from build123d import *

# Parameters (mm, degrees)
ESQUISSE7_R                  = 2.05
BOSS_EXTRU_1_DEPTH           = 8
ESQUISSE8_W                  = 8
ESQUISSE8_H                  = 5
BOSS_EXTRU_2_DEPTH           = 8
ENL_V_MAT_EXTRU_3_DEPTH      = 59.457249337
ENL_V_MAT_EXTRU_3_DEPTH_BACK = 59.457249337
ESQUISSE9_R                  = 2.05
CONG_5_R                     = 1.5


with BuildPart() as part:
    # Esquisse7 → Boss.-Extru.1 (new body)
    with BuildSketch(Plane.XY):
        with BuildLine():
            Line((0, 0), (39, 0))
            Line((39, 0), (39, 37.071067812))
            ThreePointArc((39, 37.071067812), (33.796680513, 44.858385741), (24.610912703, 43.03122292))
            Line((24.610912703, 43.03122292), (10.46877708, 28.889087297))
            ThreePointArc((10.46877708, 28.889087297), (8.641614259, 26.154544889), (8, 22.928932188))
            Line((8, 22.928932188), (8, 5))
            Line((8, 5), (0, 5))
            Line((0, 5), (0, 0))
        make_face()
        with Locations((16.428932188, 22.928932188)):
            Circle(ESQUISSE7_R, mode=Mode.SUBTRACT)
        with Locations(Location((30.571067812, 37.071067812, 0), (0, 0, 180))):
            Circle(ESQUISSE7_R, mode=Mode.SUBTRACT)
    extrude(amount=BOSS_EXTRU_1_DEPTH)

    # Esquisse8 → Boss.-Extru.2 (add)
    with BuildSketch(Plane.XY.offset(8)):
        with Locations((35, 2.5)):
            Rectangle(ESQUISSE8_W, ESQUISSE8_H)
    extrude(amount=BOSS_EXTRU_2_DEPTH)

    # Esquisse9 → Enlèv. mat.-Extru.3 (cut, two sides: drawn at the far end of the back side and taken through both)
    with BuildSketch(Plane(origin=(0, 5, 0), x_dir=(1, 0, 0), z_dir=(0, 1, 0)).offset(-ENL_V_MAT_EXTRU_3_DEPTH_BACK)):
        with Locations(Location((35, -12, 0), (0, 0, 180))):
            Circle(ESQUISSE9_R)
        with Locations(Location((4, -4, 0), (0, 0, 180))):
            Circle(ESQUISSE9_R)
    extrude(amount=ENL_V_MAT_EXTRU_3_DEPTH + ENL_V_MAT_EXTRU_3_DEPTH_BACK, mode=Mode.SUBTRACT)

    # Congé5
    cong_5_edges = [part.edges().sort_by_distance(p)[0] for p in [
        (33.796680513, 44.858385741, 0),
        (39, 18.535533906, 0),
        (0, 2.5, 0),
        (33.796680513, 44.858385741, 8),
        (17.539844892, 35.960155108, 8),
        (8.641614259, 26.154544889, 8),
        (8, 13.964466094, 8),
        (39, 21.035533906, 8),
        (31, 2.5, 16),
        (39, 2.5, 16),
        (0, 2.5, 8),
        (8, 13.964466094, 0),
        (8.641614259, 26.154544889, 0),
        (17.539844892, 35.960155108, 0),
    ]]
    fillet(cong_5_edges, radius=CONG_5_R)


solid = part.part
Work out the finished part from the listing and answer in its coordinate system (mm). A direction names the side the tool comes from. Round coordinates to 2 decimals unless told otherwise and drop trailing zeros. Loops run counter-clockwise (first coordinate to the right, second up) from the corner with the lowest first, then second, coordinate; pieces in that order, holes last. Notation, with made-up numbers: (39, 11) - (81, 11) arc R19 ccw to (81, 32) - close; hole circle Ø2 at (-27.75, 21). An arc over 180 degrees is marked (long way). Use one line per item in the form item = value. Start each with the question number.
(1) Consider line 1 (X direction, y = 2.1, z = 12); line 2 (Z direction, x = 24.5, y = 30); line 3 (X direction, y = 22, z = 4.75). Determine where each line is inside the solid, lowest interval first.
(2) Determine the mould class of faces 6 (the face through (6, 5, 3)), 7 (the face through (28.68, 37.86, 3.94)), 8 (the face through (5.627, 2.465, 2.753)), 9 (the face through (19, 0, 6)) for opening direction Y: +Y half, -Y half, draft (parallel to the pull), parting line (faces both ways), or undercut.
(3) Flat-ended cylindrical pins translate along their axes: P1, Ø4, axis at y = 11, z = 9.5, coming from the -X side; P2, Ø5, axis at y = 8, z = 11.5, coming from the +X side; P3, Ø2.5, axis at y = 2.5, z = 11, coming from the -X side; P4, Ø2, axis at x = 6.5, z = 7.5, coming from the +Y side. Find the tip coordinate at first contact, or state that the pin passes through.
(4) Which of the six approach directions +Z, -Z, +X, -X, +Y, -Y give full straight-line access (tool end or side, diameter ignored) to faces 1 (the face through (0, 3, 4)), 2 (the face through (38.55, 21.26, 7.57)), 3 (the face through (8, 14, 4)), 4 (the face through (31, 2, 11)), 5 (the face through (8.45, 13.84, 0.43))?
(5) Find section D-D on z = 12. Determine the outline of the cut face in (x, y).
(6) Find section C-C on y = 3. Determine the outline of the cut face in (x, z), and give its area (3 significant figures).
(7) Find section B-B on x = 4. Determine the outline of the cut face in (y, z).
(8) Find section A-A on z = 4. Determine the outline of the cut face in (x, y).
Answer list:
q1.line_1 = 31 to 32.95, 37.05 to 39
q1.line_2 = 0 to 8
q1.line_3 = 8 to 14.6, 18.26 to 39
q2.face_6 = +Y half
q2.face_7 = undercut
q2.face_8 = draft
q2.face_9 = -Y half
q3.P1 = 8.38
q3.P2 = through
q3.P3 = 31
q3.P4 = 5
q4.face_1 = +Z, -Z, -X, +Y, -Y
q4.face_2 = +Z, +X, +Y
q4.face_3 = +Z, -Z, -X, +Y
q4.face_4 = +Z, -X, +Y, -Y
q4.face_5 = -Z, -X, +Y
q5.outline = (31, 0) - (32.95, 0) - (32.95, 5) - (31, 5) - close; (37.05, 0) - (39, 0) - (39, 5) - (37.05, 5) - close
q6.outline = (0, 1.5) arc R1.5 ccw to (1.5, 0) - (37.5, 0) arc R1.5 ccw to (39, 1.5) - (39, 14.5) arc R1.5 ccw to (37.5, 16) - (32.5, 16) arc R1.5 ccw to (31, 14.5) - (31, 8) - (1.5, 8) arc R1.5 ccw to (0, 6.5) - close; hole circle Ø4.1 at (4, 4); hole circle Ø4.1 at (35, 12)
q6.area = 347 mm^2
q7.outline = (0, 0) - (5, 0) - (5, 1.95) - (0, 1.95) - close; (0, 6.05) - (5, 6.05) - (5, 8) - (0, 8) - close
q8.outline = (0, 0) - (1.95, 0) - (1.95, 5) - (0, 5) - close; (6.05, 0) - (39, 0) - (39, 37.07) arc R8.43 ccw to (24.61, 43.03) - (10.47, 28.89) arc R8.43 ccw to (8, 22.93) - (8, 5) - (6.05, 5) - close; hole circle Ø4.1 at (16.43, 22.93); hole circle Ø4.1 at (30.57, 37.07)
